Part print with two shaded views. Sizes in mm from the minimum x, y, z corner. A direction names the side the tool comes from. Round coordinates to 2 decimals unless told otherwise and drop trailing zeros. Loops run counter-clockwise (first coordinate to the right, second up) from the corner with the lowest first, then second, coordinate; pieces in that order, holes last. Notation, with made-up numbers: M 23,-15 L 38,-15 A32 cw 38,16 Z; hole C -14,55.25 d6. An arc over 180 degrees is marked long. Use a Markdown table: item, result. Add a question column.
Item 1: Tool access for the marked faces 4, 5, 6, 7 and 8: list every direction of +Z, -Z, +X, -X, +Y, -Y with a clear straight run to the whole face (end or side of a thin tool).
Item 2: Pin check, flat tips, straight feed: P1, Ø5, axis at x = 29.5, y = 19, coming from the +Z side; P2, Ø5.5, axis at y = 28, z = 35, coming from the +X side; P3, Ø3, axis at x = 20.5, z = 37.5, coming from the -Y side; P4, Ø2, axis at x = 13.5, z = 29, coming from the -Y side. Stop position of each tip, or through.
Item 3: Wall check: L1, parallel to Y at x = 12.1, z = 2.15; L2, parallel to Z at x = 14, y = 31; L3, parallel to Z at x = 16, y = 13.5. Give the ranges that are in metal, low to high. Write a range as from..to.
Item 4: Two-plate mould, pull along Y, no slides. Class the marked faces 1, 2 and 3: +Y half, -Y half, draft (parallel to the pull), parting line (faces both ways), or undercut.
Item 5: Saw through at C-C on y = 15. Write the cut outline in (x, z), then the cut area to 3 significant figures.
Item 6: Saw through at B-B on y = 62.04. Write the cut outline in (x, z), then the cut area to 3 significant figures.
Item 7: Saw through at D-D on z = 38.5. Write the cut outline in (x, y), then the cut area to 3 significant figures.
Item 8: Saw through at A-A on x = 17.1. Write the cut outline in (y, z).
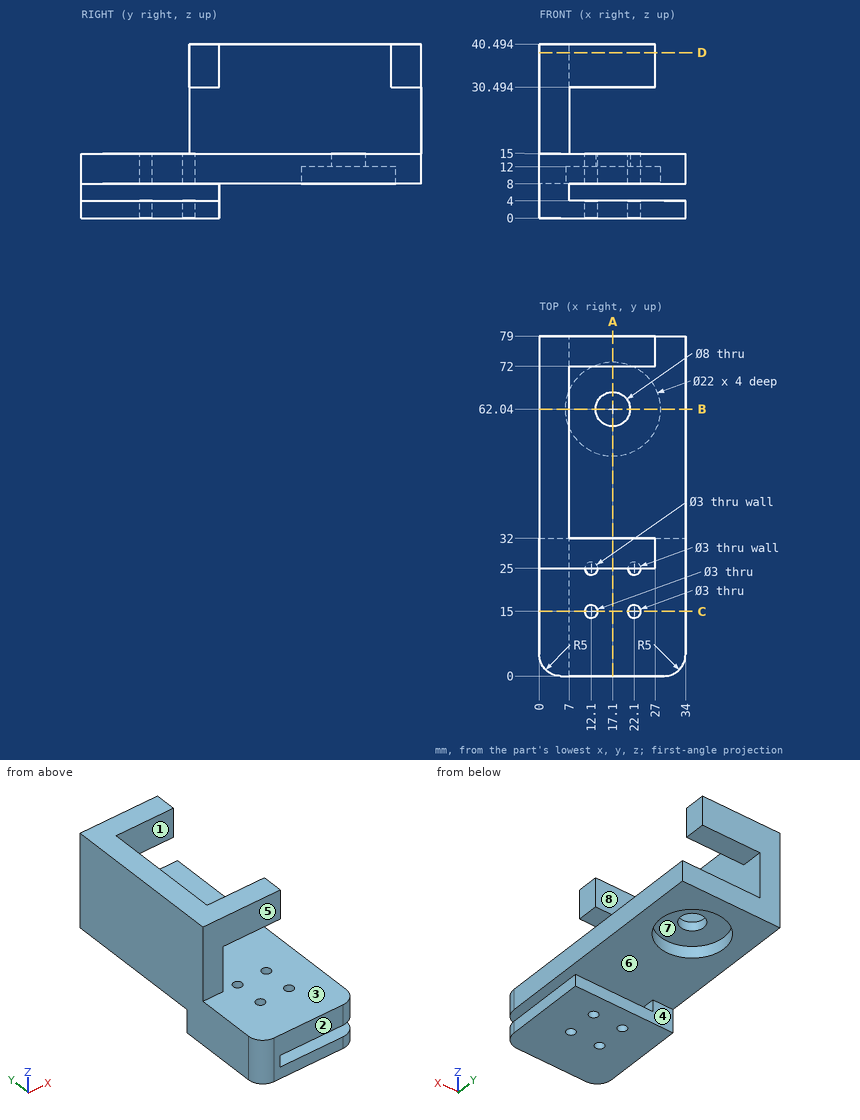
Entries:
| question | item | result |
|---|---|---|
| 1 | face 4 | -Z, +X, -X, +Y |
| 1 | face 5 | +Z, +X, -X, -Y |
| 1 | face 6 | +X, +Y |
| 1 | face 7 | -Z |
| 1 | face 8 | +Z, +X |
| 2 | P1 | z = 15 |
| 2 | P2 | x = 27 |
| 2 | P3 | y = 25 |
| 2 | P4 | through |
| 3 | L1 | 0..13.5, 16.5..23.5, 26.5..32 |
| 3 | L2 | 0..4, 8..15, 30.49..40.49 |
| 3 | L3 | 0..4, 8..15 |
| 4 | face 1 | undercut |
| 4 | face 2 | -Y half |
| 4 | face 3 | draft |
| 5 | outline | M 0,0 L 10.6,0 L 10.6,4 L 7,4 L 7,8 L 10.6,8 L 10.6,15 L 0,15 Z; M 13.6,0 L 20.6,0 L 20.6,4 L 13.6,4 Z; M 13.6,8 L 20.6,8 L 20.6,15 L 13.6,15 Z; M 23.6,0 L 34,0 L 34,4 L 23.6,4 Z; M 23.6,8 L 34,8 L 34,15 L 23.6,15 Z |
| 5 | area | 336 mm2 |
| 6 | outline | M 0,8 L 6.1,8 L 6.1,12 L 13.1,12 L 13.1,15 L 7,15 L 7,40.49 L 0,40.49 Z; M 21.1,12 L 28.1,12 L 28.1,8 L 34,8 L 34,15 L 21.1,15 Z |
| 6 | area | 304 mm2 |
| 7 | outline | M 0,25 L 27,25 L 27,32 L 7,32 L 7,72 L 27,72 L 27,79 L 0,79 Z |
| 7 | area | 658 mm2 |
| 8 | outline | M 0,0 L 32,0 L 32,4 L 0,4 Z; M 0,8 L 51.04,8 L 51.04,12 L 58.04,12 L 58.04,15 L 0,15 Z; M 25,30.49 L 32,30.49 L 32,40.49 L 25,40.49 Z; M 66.04,12 L 73.04,12 L 73.04,8 L 79,8 L 79,15 L 66.04,15 Z; M 72,30.49 L 79,30.49 L 79,40.49 L 72,40.49 Z |
